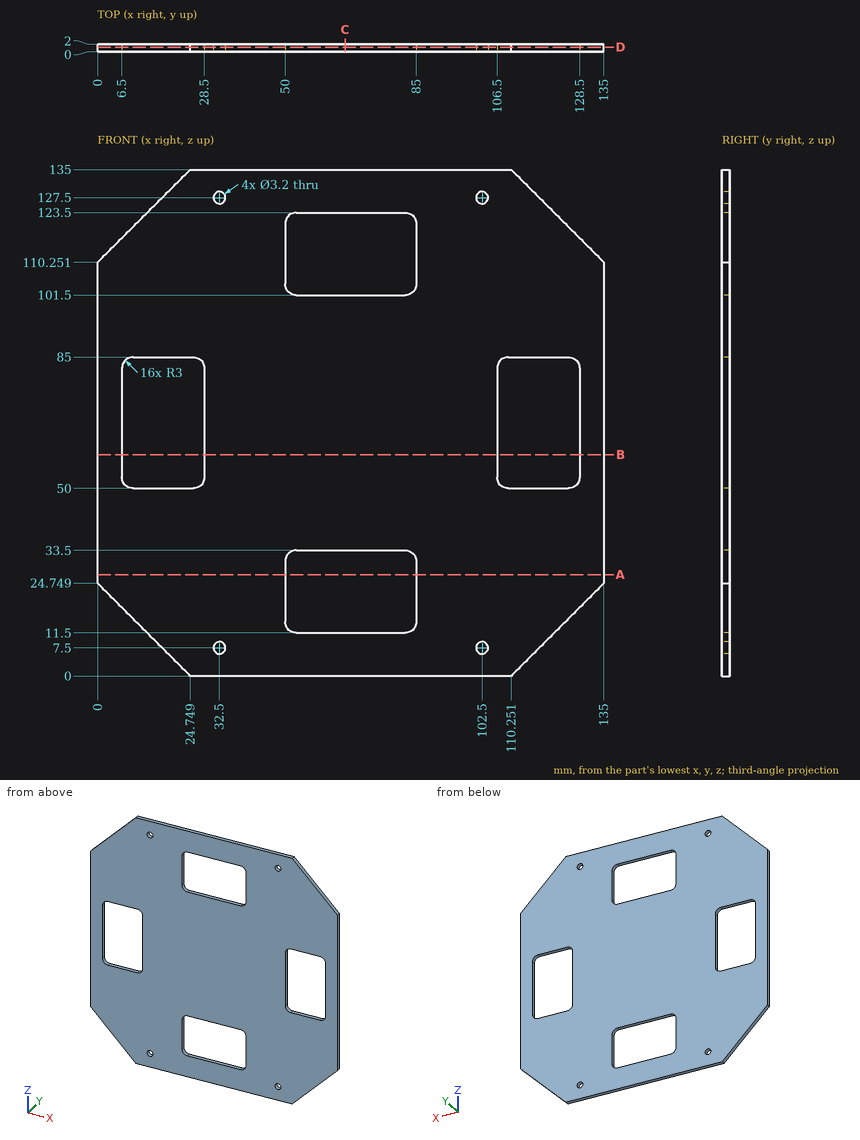
Part print with two shaded views. Sizes in mm from the minimum x, y, z corner. Give positions to 0.01 mm unless a question says otherwise; leave off trailing zeros. Write each loop counter-clockwise with the first axis right and the second up, starting at its lowest first coordinate (ties: lowest second). Pieces come first, ordered by that corner, then holes.
1) Cut at B-B on z = 59. Write the cut outline in (x, y).
Resolved:
outline: (0, 0) - (6.5, 0) - (6.5, 2) - (0, 2) - close; (28.5, 0) - (106.5, 0) - (106.5, 2) - (28.5, 2) - close; (128.5, 0) - (135, 0) - (135, 2) - (128.5, 2) - close
2) Cut at D-D on y = 1.2. State how many separate pieces and enclosed holes the cut face has, then the cut area to 3 significant figures.
Resolved:
separate pieces: 1
enclosed holes: 8
area: 13,900 mm2
3) Cut at C-C on x = 66. Write the cut outline in (y, z).
Resolved:
outline: (0, 0) - (2, 0) - (2, 11.5) - (0, 11.5) - close; (0, 33.5) - (2, 33.5) - (2, 101.5) - (0, 101.5) - close; (0, 123.5) - (2, 123.5) - (2, 135) - (0, 135) - close
4) Cut at A-A on z = 27. Write the cut outline in (x, y).
Resolved:
outline: (0, 0) - (50, 0) - (50, 2) - (0, 2) - close; (85, 0) - (135, 0) - (135, 2) - (85, 2) - close
5) Pin check, flat tips, straight feed: pin 1 (12 mm diameter, centred on x = 121, z = 117.5, fed in from -Y); pin 2 (1 mm diameter, centred on y = 1, z = 24, fed in from -X); pin 3 (1 mm diameter, centred on x = 121, y = 1, fed in from +Z); pin 4 (0.6 mm diameter, centred on x = 16, y = 1.5, fed in from +Z). Stop position of each tip, or through.
Resolved:
pin 1: stops at y = 0
pin 2: stops at x = 0.25
pin 3: stops at z = 124.75
pin 4: stops at z = 126.55
6) Probe L1, parallel to Z at x = 32.5, y = 0.7; L2, parallel to X at y = 0.3, z = 80.5; L3, parallel to X at y = 0.8, z = 7.5. List the from-to ranges inside material, lowest first.
Resolved:
L1: z = 0 to 5.9, 9.1 to 125.9, 129.1 to 135
L2: x = 0 to 6.5, 28.5 to 106.5, 128.5 to 135
L3: x = 17.25 to 30.9, 34.1 to 100.9, 104.1 to 117.75
